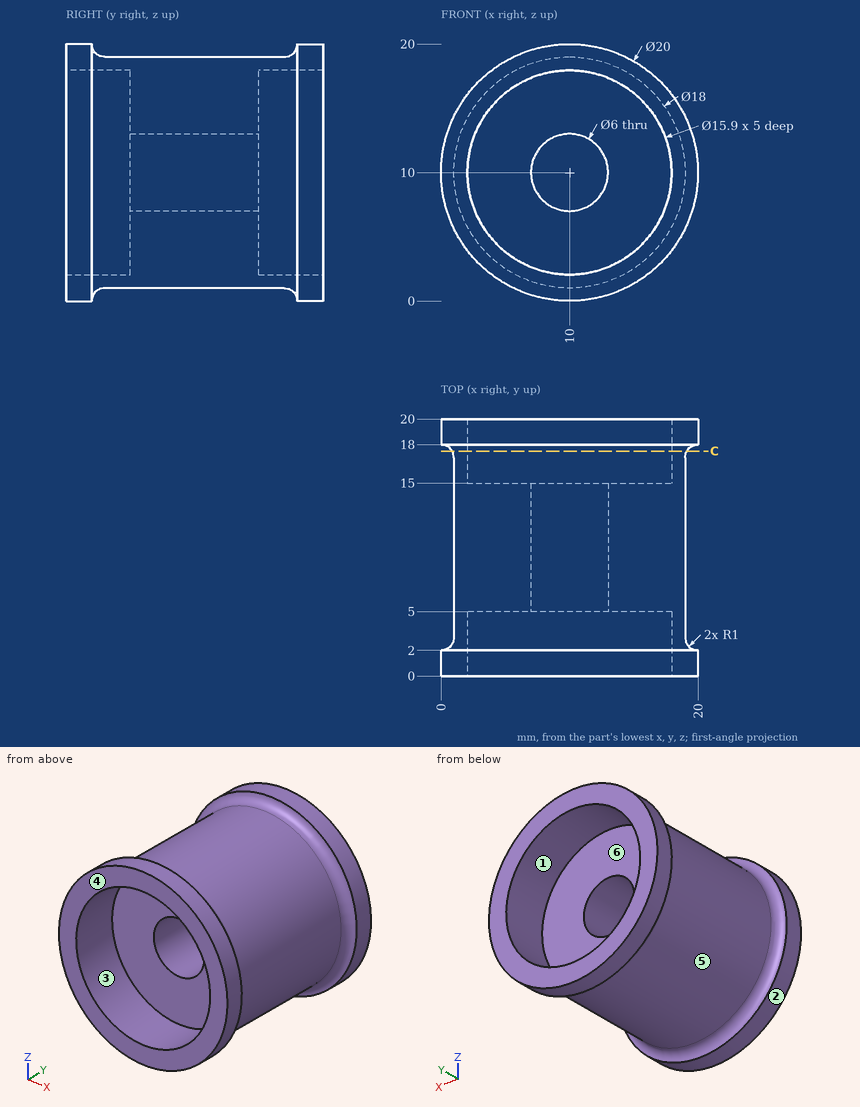
Design review of the part shown in the three views and the two pictorial views. Dimensions are in mm from the part's minimum x, y and z. A direction names the side the tool comes from. Coordinates: 2 decimals unless noted, no trailing zeros. Order: outer loops, then holes, each group sorted by start corner. A loop starts at its lowest first (then second) coordinate and runs counter-clockwise, first axis right, second up.
Item 1: Take a section at C-C, the plane y = 17.5. Write out the cut boundary in (x, z).
Item 2: For the marked faces 1, 2 and 3, list the 3-axis set-ups (+Z, -Z, +X, -X, +Y, -Y) from which the entire face can be reached by the end or side of a thin tool; tool diameter is ignored.
Item 3: The part is to be moulded in two halves that separate along X. For the marked faces 4, 5 and 6, say which applies: pulls with the +X half, pulls with the -X half, needs draft (parallel to the pull), parting line crosses it, or undercut.
Item 4: For pin 1 Ø8 at (x, z) = (10, 10.5) entering from -Y; pin 2 Ø9.5 at (x, z) = (10, 10) entering from +Y; pin 3 Ø3 at (y, z) = (5, 3.5) entering from +X, all flat-tipped, find the tip position at first contact; note any pin that passes through.
Item 5: For line 1 (X direction, y = 16.7, z = 10); line 2 (X direction, y = 8.75, z = 10); line 3 (Z direction, x = 7.5, y = 3.75), list the stretches that pass through material, from the lowest coordinate up.
The answers:
1. outline: circle Ø18.27 at (10, 10); hole circle Ø15.9 at (10, 10)
2. face 1: +Y
2. face 2: +Y, -Y
2. face 3: -Y
3. face 4: needs draft
3. face 5: parting line crosses it
3. face 6: undercut
4. pin 1: stops at y = 5
4. pin 2: stops at y = 15
4. pin 3: stops at x = 17.48
5. line 1: x = 1 to 2.05, 17.95 to 19
5. line 2: x = 1 to 7, 13 to 19
5. line 3: z = 1.35 to 2.45, 17.55 to 18.65
